from build123d import *

# Parameters (mm, degrees)
SKETCH_1_R      = 1.5
SKETCH_1_R_2    = 4
EXTRUDE_1_DEPTH = 4


with BuildPart() as part:
    # 草图1 → 凸台-拉伸1 (new body)
    with BuildSketch(Plane.XY):
        with BuildLine():
            Line((-4, 16.63598728), (-9.255774721, 3.785582428))
            ThreePointArc((-9.255774721, 3.785582428), (0, -10), (9.255774721, 3.785582428))
            Line((9.255774721, 3.785582428), (4, 16.63598728))
            ThreePointArc((4, 16.63598728), (0, 19.321626358), (-4, 16.63598728))
        make_face()
        with Locations((-7, 0)):
            Circle(SKETCH_1_R, mode=Mode.SUBTRACT)
        with Locations((7, 0)):
            Circle(SKETCH_1_R, mode=Mode.SUBTRACT)
        with Locations((0, -7)):
            Circle(SKETCH_1_R, mode=Mode.SUBTRACT)
        with Locations((0, 13)):
            Circle(SKETCH_1_R, mode=Mode.SUBTRACT)
        Circle(SKETCH_1_R_2, mode=Mode.SUBTRACT)
    extrude(amount=EXTRUDE_1_DEPTH)


solid = part.part
Input: part model. Units: mm. Frame: model coordinates. Round coordinates to 2 decimals unless told otherwise and drop trailing zeros. Order: outer loops, then holes, each group sorted by start corner. A loop starts at its lowest first (then second) coordinate and runs counter-clockwise, first axis right, second up.
1. Cut plane C-C, the plane z = 2.95. Output: boundary loops of the cut face in (x, y), then the cut area to 3 significant figures.
The answers:
outline: (-9.26, 3.79) arc R10 ccw (long way) to (9.26, 3.79) - (4, 16.64) arc R4.32 ccw to (-4, 16.64) - close; hole circle Ø3 at (-7, 0); hole circle Ø8 at (0, 0); hole circle Ø3 at (0, -7); hole circle Ø3 at (0, 13); hole circle Ø3 at (7, 0)
area: 338 mm2
2. Mould query, pull axis X, two halves, no side actions, for faces 1 (the face through (0, 5, 0)), 2 (the face through (6.665, 10.121, 1.972)), 3 (the face through (-0.325, -8.464, 1.972)), 4 (the face through (-0.325, 11.536, 1.972)). Classes: released by +X, released by -X, zero draft, split by the parting line, or undercut.
The answers:
face 1: zero draft
face 2: released by +X
face 3: undercut
face 4: undercut
3. Cut plane B-B, the plane x = 0. Output: boundary loops of the cut face in (y, z).
The answers:
outline: (-10, 0) - (-8.5, 0) - (-8.5, 4) - (-10, 4) - close; (-5.5, 0) - (-4, 0) - (-4, 4) - (-5.5, 4) - close; (4, 0) - (11.5, 0) - (11.5, 4) - (4, 4) - close; (14.5, 0) - (19.32, 0) - (19.32, 4) - (14.5, 4) - close
4. Cut plane A-A, the plane y = 0. Output: boundary loops of the cut face in (x, z), then the cut area to 3 significant figures.
The answers:
outline: (-10, 0) - (-8.5, 0) - (-8.5, 4) - (-10, 4) - close; (-5.5, 0) - (-4, 0) - (-4, 4) - (-5.5, 4) - close; (4, 0) - (5.5, 0) - (5.5, 4) - (4, 4) - close; (8.5, 0) - (10, 0) - (10, 4) - (8.5, 4) - close
area: 24.0 mm2
5. Cut plane D-D, the plane x = 7. Output: boundary loops of the cut face in (y, z).
The answers:
outline: (-7.14, 0) - (-1.5, 0) - (-1.5, 4) - (-7.14, 4) - close; (1.5, 0) - (9.3, 0) - (9.3, 4) - (1.5, 4) - close
6. Pin query (flat end, axial travel): P1, Ø2.5, axis at x = 0, y = 13, coming from the +Z side; P2, Ø3.5, axis at x = -7, y = 0, coming from the -Z side; P3, Ø2, axis at x = 5, z = 2, coming from the +Y side; P4, Ø1.5, axis at x = -6, z = 0.5, coming from the -Y side. Return the tip coordinate at first contact, or that it passes through.
The answers:
P1: passes through
P2: stops at z = 0
P3: stops at y = 16.64
P4: stops at y = -8.51
7. Material intervals for line 1 (Y direction, x = 0, z = 1.75); line 2 (Y direction, x = -1, z = 0.75); line 3 (Y direction, x = 7, z = 2.5), sorted ascending.
The answers:
line 1: y = -10 to -8.5, -5.5 to -4, 4 to 11.5, 14.5 to 19.32
line 2: y = -9.95 to -8.12, -5.88 to -3.87, 3.87 to 11.88, 14.12 to 19.2
line 3: y = -7.14 to -1.5, 1.5 to 9.3
